from build123d import *

# Parameters (mm, degrees)
BOSS_EXTRUDE1_DEPTH = 13
SKETCH5_W           = 154.5
SKETCH5_H           = 154.5
CUT_EXTRUDE3_DEPTH  = 12
CUT_EXTRUDE4_DEPTH  = 11
SKETCH8_W           = 5
SKETCH8_H           = 10
BOSS_EXTRUDE2_DEPTH = 2
SKETCH9_W           = 10
SKETCH9_H           = 5
BOSS_EXTRUDE3_DEPTH = 2
SKETCH11_W          = 10
SKETCH11_H          = 4.300504792
BOSS_EXTRUDE4_DEPTH = 2


with BuildPart() as part:
    # Sketch1 → Boss-Extrude1 (new body)
    with BuildSketch(Plane(origin=(0, 0, 0), x_dir=(1, 0, 0), z_dir=(0, 1, 0))):
        Polygon((20, 158.5), (0, 138.5), (0, 20), (20, 0), (138.5, 0), (158.5, 20), (158.5, 138.5), (138.5, 158.5), align=None)
    extrude(amount=BOSS_EXTRUDE1_DEPTH)

    # Sketch5 → Cut-Extrude3 (cut)
    with BuildSketch(Plane.XZ):
        with Locations((79.25, -79.25)):
            Rectangle(SKETCH5_W, SKETCH5_H)
    extrude(amount=-CUT_EXTRUDE3_DEPTH, mode=Mode.SUBTRACT)

    # Sketch7 → Cut-Extrude4 (cut)
    with BuildSketch(Plane(origin=(0, 13, 0), x_dir=(1, 0, 0), z_dir=(0, 1, 0))):
        Polygon((138.5, 122.726497308), (138.5, 134.273502692), (128.5, 140.047005384), (118.5, 134.273502692), (118.5, 122.726497308), (128.5, 116.952994616), align=None)
        Polygon((105.5, 122.726497308), (105.5, 134.273502692), (95.5, 140.047005384), (85.5, 134.273502692), (85.5, 122.726497308), (95.5, 116.952994616), align=None)
        Polygon((72.5, 122.726497308), (72.5, 134.273502692), (62.5, 140.047005384), (52.5, 134.273502692), (52.5, 122.726497308), (62.5, 116.952994616), align=None)
        Polygon((39.5, 122.726497308), (39.5, 134.273502692), (29.5, 140.047005384), (19.5, 134.273502692), (19.5, 122.726497308), (29.5, 116.952994616), align=None)
        Polygon((105.5, 89.726497308), (105.5, 101.273502692), (95.5, 107.047005384), (85.5, 101.273502692), (85.5, 89.726497308), (95.5, 83.952994616), align=None)
        Polygon((72.5, 89.726497308), (72.5, 101.273502692), (62.5, 107.047005384), (52.5, 101.273502692), (52.5, 89.726497308), (62.5, 83.952994616), align=None)
        Polygon((39.5, 89.726497308), (39.5, 101.273502692), (29.5, 107.047005384), (19.5, 101.273502692), (19.5, 89.726497308), (29.5, 83.952994616), align=None)
        Polygon((105.5, 56.726497308), (105.5, 68.273502692), (95.5, 74.047005384), (85.5, 68.273502692), (85.5, 56.726497308), (95.5, 50.952994616), align=None)
        Polygon((72.5, 56.726497308), (72.5, 68.273502692), (62.5, 74.047005384), (52.5, 68.273502692), (52.5, 56.726497308), (62.5, 50.952994616), align=None)
        Polygon((39.5, 56.726497308), (39.5, 68.273502692), (29.5, 74.047005384), (19.5, 68.273502692), (19.5, 56.726497308), (29.5, 50.952994616), align=None)
        Polygon((105.5, 23.726497308), (105.5, 35.273502692), (95.5, 41.047005384), (85.5, 35.273502692), (85.5, 23.726497308), (95.5, 17.952994616), align=None)
        Polygon((72.5, 23.726497308), (72.5, 35.273502692), (62.5, 41.047005384), (52.5, 35.273502692), (52.5, 23.726497308), (62.5, 17.952994616), align=None)
        Polygon((39.5, 23.726497308), (39.5, 35.273502692), (29.5, 41.047005384), (19.5, 35.273502692), (19.5, 23.726497308), (29.5, 17.952994616), align=None)
        Polygon((138.5, 89.726497308), (138.5, 101.273502692), (128.5, 107.047005384), (118.5, 101.273502692), (118.5, 89.726497308), (128.5, 83.952994616), align=None)
        Polygon((138.5, 56.726497308), (138.5, 68.273502692), (128.5, 74.047005384), (118.5, 68.273502692), (118.5, 56.726497308), (128.5, 50.952994616), align=None)
        Polygon((138.5, 23.726497308), (138.5, 35.273502692), (128.5, 41.047005384), (118.5, 35.273502692), (118.5, 23.726497308), (128.5, 17.952994616), align=None)
    extrude(amount=-CUT_EXTRUDE4_DEPTH, mode=Mode.SUBTRACT)

    # Sketch8 → Boss-Extrude2 (add)
    with BuildSketch(Plane.XZ):
        with Locations((2.5, -34.05439508)):
            Rectangle(SKETCH8_W, SKETCH8_H)
        with Locations((2.5, -124.44560492)):
            Rectangle(SKETCH8_W, SKETCH8_H)
        with Locations((156, -124.44560492)):
            Rectangle(SKETCH8_W, SKETCH8_H)
        with Locations((156, -34.05439508)):
            Rectangle(SKETCH8_W, SKETCH8_H)
    extrude(amount=BOSS_EXTRUDE2_DEPTH)

    # Sketch9 → Boss-Extrude3 (add)
    with BuildSketch(Plane(origin=(5, 0, 0), x_dir=(0, 0, -1), z_dir=(1, 0, 0))):
        with Locations((124.44560492, 0.5)):
            Rectangle(SKETCH9_W, SKETCH9_H)
        with Locations((34.05439508, 0.5)):
            Rectangle(SKETCH9_W, SKETCH9_H)
    extrude(amount=BOSS_EXTRUDE3_DEPTH)

    # Sketch11 → Boss-Extrude4 (add)
    with BuildSketch(Plane.ZY.offset(-153.5)):
        with Locations((-124.44560492, 0.150252396)):
            Rectangle(SKETCH11_W, SKETCH11_H)
        with Locations((-34.05439508, 0.150252396)):
            Rectangle(SKETCH11_W, SKETCH11_H)
    extrude(amount=BOSS_EXTRUDE4_DEPTH)


solid = part.part
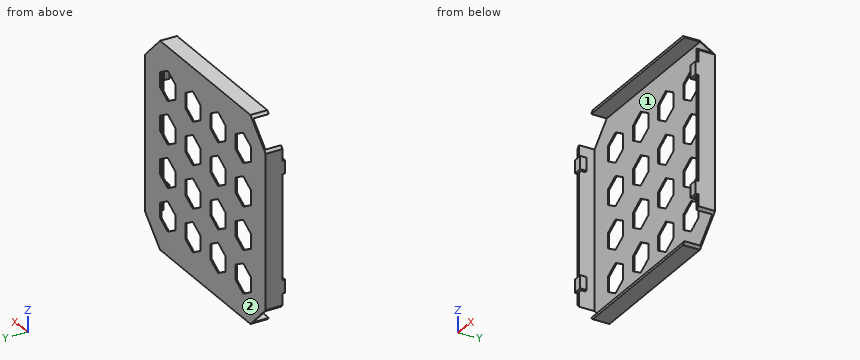
Geometry check sheet. Reference: the model listing, model coordinates, mm. Face numbers are marked on the shaded views. Coordinates: 2 decimals unless noted, no trailing zeros. Order: outer loops, then holes, each group sorted by start corner. A loop starts at its lowest first (then second) coordinate and runs counter-clockwise, first axis right, second up. Notation, with made-up numbers: M 75.5,21.5 L 117.5,21.5 A12 cw 117.5,37.5 Z; hole C 84,15 d5. An arc over 180 degrees is marked long. Use CSV: the item, a comma, the result in double quotes.
Item 1: Cross-section at C-C on y = 8.5. Record the cut outline in (x, z).
Returned:
outline,"M 0,-138.5 L 2,-140.5 L 2,-18 L 0,-20 Z; M 18,-156.5 L 20,-158.5 L 138.5,-158.5 L 140.5,-156.5 Z; M 18,-2 L 140.5,-2 L 138.5,0 L 20,0 Z; M 156.5,-140.5 L 158.5,-138.5 L 158.5,-20 L 156.5,-18 Z"
Item 2: Cross-section at A-A on z = -94. Record the cut outline in (x, y), then the cut area to 4 significant figures.
Returned:
outline,"M 0,0 L 2,0 L 2,12 L 19.5,12 L 19.5,13 L 0,13 Z; M 39.5,12 L 52.5,12 L 52.5,13 L 39.5,13 Z; M 72.5,12 L 85.5,12 L 85.5,13 L 72.5,13 Z; M 105.5,12 L 118.5,12 L 118.5,13 L 105.5,13 Z; M 138.5,12 L 156.5,12 L 156.5,0 L 158.5,0 L 158.5,13 L 138.5,13 Z"
area,"126.5 mm2"
Item 3: Thickness scan on line 1 along X through (y, z) = (2.5, -124.5); line 2 along Z through (x, y) = (41.5, 2.5); line 3 along X through (y, z) = (4.75, -88). Record the ranges inside material, lowest first.
Returned:
line 1,"x = 0 to 2, 5 to 7, 156.5 to 158.5"
line 2,"z = -158.5 to -156.5, -2 to 0"
line 3,"x = 0 to 2, 156.5 to 158.5"
Item 4: Cross-section at B-B on x = 36.5. Record the cut outline in (y, z), then the cut area to 3 significant figures.
Returned:
outline,"M 0,-158.5 L 13,-158.5 L 13,-136.01 L 12,-136.01 L 12,-156.5 L 0,-156.5 Z; M 0,-2 L 12,-2 L 12,-21.99 L 13,-21.99 L 13,0 L 0,0 Z; M 12,-120.99 L 13,-120.99 L 13,-103.01 L 12,-103.01 Z; M 12,-87.99 L 13,-87.99 L 13,-70.01 L 12,-70.01 Z; M 12,-54.99 L 13,-54.99 L 13,-37.01 L 12,-37.01 Z"
area,"146 mm2"
Item 5: Cross-section at D-D on z = -77. Record the cut outline in (x, y), then the cut area to 4 significant figures.
Returned:
outline,"M 0,0 L 2,0 L 2,12 L 156.5,12 L 156.5,0 L 158.5,0 L 158.5,13 L 0,13 Z"
area,"206.5 mm2"
Item 6: Gauge pin test, flat ends, axial feed: pin 1 Ø10 at (x, z) = (111.5, -38.5) entering from -Y; pin 2 Ø2 at (x, z) = (157.5, -24) entering from -Y; pin 3 Ø1 at (x, y) = (140.5, 9) entering from +Z. Record the tip position at first contact, or that the pin passes through.
Returned:
pin 1,"stops at y = 12"
pin 2,"stops at y = 0"
pin 3,"stops at z = -1.5"
Item 7: Mould release check, pull along Z, two halves, no side actions. Record for the marked faces 1 and 2: pulls with the +Z half, pulls with the -Z half, needs draft (parallel to the pull), parting line crosses it, or undercut.
Returned:
face 1,"undercut"
face 2,"needs draft"
